```python
from build123d import *

# Parameters (mm, degrees)
EXTRUDE_1_DEPTH     = 5
SKETCH_2_R          = 1.7
EXTRUDE_2_DEPTH     = 6
SKETCH_3_R          = 1.7
CUT_EXTRUDE_1_DEPTH = 4


with BuildPart() as part:
    # 草图1 → 凸台-拉伸1 (new body)
    with BuildSketch(Plane(origin=(0, 0, 0), x_dir=(1, 0, 0), z_dir=(0, 1, 0))):
        Polygon((1.3125, -2.273316685), (2.625, 0), (1.3125, 2.273316685), (-1.3125, 2.273316685), (-2.625, 0), (-1.3125, -2.273316685), align=None)
    extrude(amount=EXTRUDE_1_DEPTH)

    # 草图2 → 凸台-拉伸2 (add)
    with BuildSketch(Plane(origin=(0, 0, 0), x_dir=(1, 0, 0), z_dir=(0, 1, 0))):
        with Locations(Location((0, 0, 0), (0, 0, 270))):
            Circle(SKETCH_2_R)
    extrude(amount=-EXTRUDE_2_DEPTH)

    # 草图3 → 切除-拉伸1 (cut)
    with BuildSketch(Plane(origin=(0, 5, 0), x_dir=(1, 0, 0), z_dir=(0, 1, 0))):
        with Locations(Location((0, 0, 0), (0, 0, 270))):
            Circle(SKETCH_3_R)
    extrude(amount=-CUT_EXTRUDE_1_DEPTH, mode=Mode.SUBTRACT)


solid = part.part
```
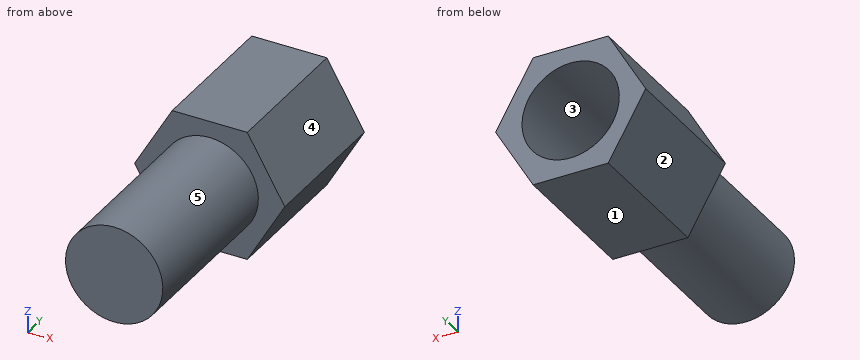
Check sheet for the modelled part. Datum: model origin and axes. Units: mm. Face numbers are marked on the shaded views. A direction names the side the tool comes from. Coordinates: 2 decimals unless noted, no trailing zeros. Loops run counter-clockwise (first coordinate to the right, second up) from the corner with the lowest first, then second, coordinate; pieces in that order, holes last.
1) Material ranges on probe 1 along Y at (x, z) = (0.15, 0.9); probe 2 along X at (y, z) = (1.5, -1.35); probe 3 along X at (y, z) = (2.5, 0.95), recorded low to high.
2) Gauge pin test, flat end, axial feed: pin 1 (2 mm diameter, centred on y = -3.5, z = -0.5, fed in from -X). Record the tip position at first contact, or that the pin passes through.
3) Access from +Z, -Z, +X, -X, +Y, -Y to the whole of each face (thin tool, end or side, straight path). Record for the marked faces 4 and 5.
4) Sectioned sample at B-B (x = 0). Record the boundary of the cut face in (y, z), and give its area (3 significant figures).
5) Release check for a two-part mould opening along X. For the marked faces 1, 2 and 3 record: released by +X, released by -X, zero draft, split by the parting line, or undercut.
6) Sectioned sample at A-A (y = 3.25). Record the boundary of the cut face in (x, z) (1 decimal), and give its area (3 significant figures).
7) Sectioned sample at C-C (z = 0.6). Record the boundary of the cut face in (x, y), and give its area (3 significant figures).
8) Sectioned sample at D-D (y = -1). Record the boundary of the cut face in (x, z), and give its area (3 significant figures).
Check sheet entries:
1. probe 1: y = -6 to 1
1. probe 2: x = -1.85 to -1.03, 1.03 to 1.85
1. probe 3: x = -2.08 to -1.41, 1.41 to 2.08
2. pin 1: stops at x = -1.7
3. face 4: +Z, +X, +Y, -Y
3. face 5: -Y
4. outline: (-6, -1.7) - (0, -1.7) - (0, -2.27) - (5, -2.27) - (5, -1.7) - (1, -1.7) - (1, 1.7) - (5, 1.7) - (5, 2.27) - (0, 2.27) - (0, 1.7) - (-6, 1.7) - close
4. area: 29.5 mm2
5. face 1: zero draft
5. face 2: released by -X
5. face 3: undercut
6. outline: (-2.6, 0) - (-1.3, -2.3) - (1.3, -2.3) - (2.6, 0) - (1.3, 2.3) - (-1.3, 2.3) - close; hole circle Ø3.4 at (0, 0)
6. area: 8.82 mm2
7. outline: (-2.28, 0) - (-1.59, 0) - (-1.59, -6) - (1.59, -6) - (1.59, 0) - (2.28, 0) - (2.28, 5) - (1.59, 5) - (1.59, 1) - (-1.59, 1) - (-1.59, 5) - (-2.28, 5) - close
7. area: 29.1 mm2
8. outline: circle Ø3.4 at (0, 0)
8. area: 9.08 mm2
